Here's how the part is built. I have some questions about the finished solid (model axes, mm). A direction names the side the tool comes from. Give positions to 0.01 mm unless a question says otherwise; leave off trailing zeros. Loops run counter-clockwise (first coordinate to the right, second up) from the corner with the lowest first, then second, coordinate; pieces in that order, holes last. Notation, with made-up numbers: (0, 80) - (4, 80) arc R22 ccw to (4, 90) - close; hole circle Ø4 at (-20, -26). An arc over 180 degrees is marked (long way). Use one line per item in the form item = value.
from build123d import *

# Parameters (mm, degrees)
SKETCH_1_W             = 100
SKETCH_1_H             = 70
EXTRUDE_1_DEPTH        = 30
SKETCH_2_W             = 18
SKETCH_2_H             = 60
CUT_EXTRUDE_1_DEPTH    = 58
HOLE_WIZARD_9_0_9_1_D  = 9
CUT_EXTRUDE_2_REACH    = 87.586
HOLE_WIZARD_8_0_8_1_D  = 8
HOLE_WIZARD_M5_1_D     = 4.2
HOLE_WIZARD_M5_1_DEPTH = 16
HOLE_WIZARD_M5_1_TIP   = 1.2618073
CHAMFER_1_SIZE         = 2


with BuildPart() as part:
    # 草圖1 → 伸長1 (new, symmetric)
    with BuildSketch(Plane.XY):
        Rectangle(SKETCH_1_W, SKETCH_1_H)
    extrude(amount=EXTRUDE_1_DEPTH, both=True)

    # 草圖2 → 除料-伸長1 (cut)
    with BuildSketch(Plane(origin=(0, 35, 0), x_dir=(1, 0, 0), z_dir=(0, 1, 0))):
        with Locations((41, 0)):
            Rectangle(SKETCH_2_W, SKETCH_2_H)
        with Locations((-41, 0)):
            Rectangle(SKETCH_2_W, SKETCH_2_H)
    extrude(amount=-CUT_EXTRUDE_1_DEPTH, mode=Mode.SUBTRACT)

    # Ø9.0 (9) 直徑孔1 (through all)
    with Locations(Plane(origin=(-40, -23, 55), x_dir=(-1, 0, 0), z_dir=(0, 1, 0))):
        with Locations((0, -75), (-80, -75), (-80, -35), (0, -35)):
            Hole(HOLE_WIZARD_9_0_9_1_D / 2)

    # 草圖17 → 除料-伸長2 (cut, up to next)
    with BuildSketch(Plane(origin=(0, 0, -30), x_dir=(-1, 0, 0), z_dir=(0, 0, -1)), mode=Mode.PRIVATE) as cut_extrude_2_sk1:
        with BuildLine():
            Line((13, -23), (-13, -23))
            ThreePointArc((-13, -23), (-13.707106781, -22.707106781), (-14, -22))
            Line((-14, -22), (-14, 28))
            ThreePointArc((-14, 28), (-13.707106781, 28.707106781), (-13, 29))
            Line((-13, 29), (13, 29))
            ThreePointArc((13, 29), (13.707106781, 28.707106781), (14, 28))
            Line((14, 28), (14, -22))
            ThreePointArc((14, -22), (13.707106781, -22.707106781), (13, -23))
        make_face()
    cut_extrude_2_tool1 = extrude(cut_extrude_2_sk1.sketch, amount=-CUT_EXTRUDE_2_REACH, mode=Mode.PRIVATE) & part.part
    add(cut_extrude_2_tool1.solids().sort_by_distance((0, 3, -30))[0], mode=Mode.SUBTRACT)

    # Ø8.0 (8) 直徑孔1 (through all)
    with Locations(Plane(origin=(20, -23, 5.325436893), x_dir=(-1, 0, 0), z_dir=(0, 1, 0))):
        with Locations((60, -5.325436893), (-20, -5.325436893)):
            Hole(HOLE_WIZARD_8_0_8_1_D / 2)

    # M5 螺紋孔1
    with Locations(Plane(origin=(0, 35, 0), x_dir=(-1, 0, 0), z_dir=(0, 1, 0))):
        with Locations((25, 17.4), (-25, 17.4), (-25, -2.6), (25, -2.6)):
            Hole(HOLE_WIZARD_M5_1_D / 2, depth=HOLE_WIZARD_M5_1_DEPTH)
            with Locations((0, 0, -(HOLE_WIZARD_M5_1_DEPTH + HOLE_WIZARD_M5_1_TIP / 2))):  # 118° drill point
                Cone(0, HOLE_WIZARD_M5_1_D / 2, HOLE_WIZARD_M5_1_TIP, mode=Mode.SUBTRACT)

    # 導角1
    chamfer_1_edges = [part.edges().sort_by_distance(p)[0] for p in [
        (50, -29, 30),
        (32, 35, 0),
        (-50, -29, -30),
        (-50, -29, 30),
        (-32, 35, 0),
        (50, -29, -30),
    ]]
    chamfer(chamfer_1_edges, length=CHAMFER_1_SIZE)


solid = part.part
(1) If we section it at A-A (x = 40): List the corners of the cut face in (y, z) for me, plus the area to 3 significant figures.
Geometry says:
outline = (-35, -30) - (-23, -30) - (-23, -24.5) - (-35, -24.5) - close; (-35, -15.5) - (-23, -15.5) - (-23, -4) - (-35, -4) - close; (-35, 4) - (-23, 4) - (-23, 15.5) - (-35, 15.5) - close; (-35, 24.5) - (-23, 24.5) - (-23, 30) - (-35, 30) - close
area = 408 mm²
(2) If I drill on probe 1 along X at (y, z) = (23.25, 17.4); probe 2 along Z at (x, y) = (-40, -31.25); probe 3 along X at (y, z) = (31.25, -2.6), over which ranges is the centre line in solid material (lowest first)?
Geometry says:
probe_1 = -32 to -27.1, -22.9 to -14, 14 to 22.9, 27.1 to 32
probe_2 = -30 to -24.5, -15.5 to -4, 4 to 15.5, 24.5 to 30
probe_3 = -32 to -27.1, -22.9 to 22.9, 27.1 to 32
(3) If we section it at B-B (y = -5): List the corners of the cut face in (x, z) for me, plus the area to 3 significant figures.
Geometry says:
outline = (-32, -30) - (-14, -30) - (-14, 30) - (-32, 30) - close; (14, -30) - (32, -30) - (32, 30) - (14, 30) - close
area = 2,160 mm²
(4) For P1, Ø15, axis at y = 15, z = -3, coming from the -X side; P2, Ø2, axis at y = 1, z = -20, coming from the +X side; P3, Ø20, axis at x = -44, z = -7.5, coming from the +Y side, each with a flat end and sliding along its axis, tell me the tip position at first contact or that it passes through.
Geometry says:
P1 = -32
P2 = 32
P3 = -23
(5) If we section it at D-D (x = 0.5): List the corners of the cut face in (y, z) for me.
Geometry says:
outline = (-35, -30) - (-23, -30) - (-23, 30) - (-35, 30) - close; (29, -30) - (35, -30) - (35, 30) - (29, 30) - close
(6) If we section it at C-C (z = -20): List the corners of the cut face in (x, y) for me.
Geometry says:
outline = (-50, -35) - (-44.5, -35) - (-44.5, -23) - (-50, -23) - close; (-35.5, -35) - (35.5, -35) - (35.5, -23) - (32, -23) - (32, 33) - (30, 35) - (-30, 35) - (-32, 33) - (-32, -23) - (-35.5, -23) - close; (44.5, -35) - (50, -35) - (50, -23) - (44.5, -23) - close; hole (-14, -22) arc R1 ccw to (-13, -23) - (13, -23) arc R1 ccw to (14, -22) - (14, 28) arc R1 ccw to (13, 29) - (-13, 29) arc R1 ccw to (-14, 28) - close
(7) For faces 5 (the flat face through (0, 29, 0)), 6 (the flat face through (-45, -23, 0)), 7 (the cylindrical face through (27.003, 26.888, -1.969)), 8 (the flat face through (-50, -29, 0)), which set-ups out of +Z, -Z, +X, -X, +Y, -Y let a thin tool reach every point of the face, with its end or its side?
Geometry says:
face_5 = +Z, -Z
face_6 = +Z, -Z, -X, +Y
face_7 = +Y
face_8 = +Z, -Z, -X, +Y, -Y
(8) Thinking about a two-plate mould opening in X: for faces 1 (the flat face through (32, 5, 0)), 2 (the cylindrical face through (25.969, 26.888, 15.537)), 3 (the flat face through (0, -23, 0)), 4 (the flat face through (-1, -35, 0)), which applies, pulls with the +X half, pulls with the -X half, needs draft (parallel to the pull), parting line crosses it, or undercut?
Geometry says:
face_1 = pulls with the +X half
face_2 = undercut
face_3 = undercut
face_4 = needs draft
